```python
from build123d import *

# Parameters (mm, degrees)
BOSS_EXTRUDE1_DEPTH = 21
CHAMFER1_SIZE       = 0.5


with BuildPart() as part:
    # Sketch1 → Boss-Extrude1 (new body)
    with BuildSketch(Plane(origin=(0, 0, 0), x_dir=(1, 0, 0), z_dir=(0, 1, 0))):
        Polygon((4.041451884, 0), (2.020725942, 3.5), (-2.020725942, 3.5), (-4.041451884, 0), (-2.020725942, -3.5), (2.020725942, -3.5), align=None)
    extrude(amount=BOSS_EXTRUDE1_DEPTH)

    # Sketch2 → Cut-Revolve1 (revolve, cut)
    with BuildSketch(Plane.XY, mode=Mode.PRIVATE) as cut_revolve1_sk:
        Polygon((-1, 1.985640646), (-1, 21.445867252), (0, 21.445867252), (0, 0), (-0.2, 0), (-0.2, 0.6), align=None)
        Polygon((-3, 22.847292178), (-3, 6.770566956), (-2.5, 6.5), (-2.5, 5), (-6.012196156, 5), (-6.012196156, 2), (-1.654700538, 2), (-0.5, 0), (-0.5, -1.473098258), (-7.184398373, -1.473098258), (-7.184398373, 22.847292178), align=None)
    revolve(cut_revolve1_sk.sketch.rotate(Axis((0, 22.126511162, 0), (0, -1, 0)), 270), axis=Axis((0, 22.126511162, 0), (0, -1, 0)), mode=Mode.SUBTRACT)

    # Chamfer1
    chamfer1_edges = [part.edges().sort_by_distance(p)[0] for p in [
        (0, 21, -1),
        (0, 21, -3),
    ]]
    chamfer(chamfer1_edges, length=CHAMFER1_SIZE)


solid = part.part
```
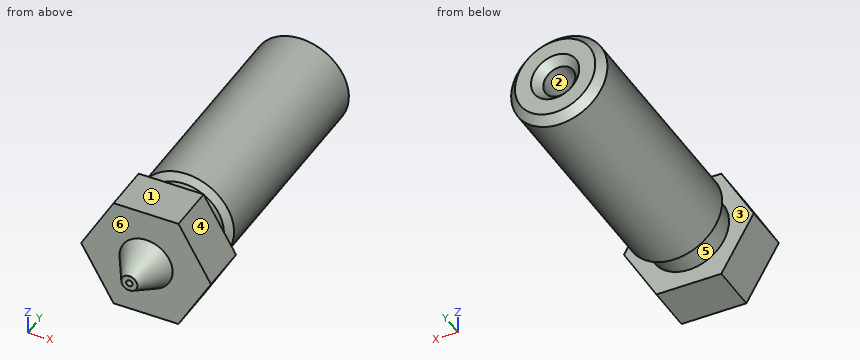
Could you check a few things on this model? Use its own coordinates, in mm. Face numbers are marked on the shaded views. A direction names the side the tool comes from. Round coordinates to 2 decimals unless told otherwise and drop trailing zeros. Write each loop counter-clockwise with the first axis right and the second up, starting at its lowest first coordinate (ties: lowest second). Pieces come first, ordered by that corner, then holes.
(1) Suppose I cut it at A-A on x = 0. Write out the boundary of the cut face in (y, z), and give its area (3 significant figures).
Findings below:
outline: (0, -0.5) - (2, -1.65) - (2, -3.5) - (5, -3.5) - (5, -2.5) - (6.5, -2.5) - (6.77, -3) - (20.5, -3) - (21, -2.5) - (21, -1.5) - (20.5, -1) - (1.99, -1) - (0.6, -0.2) - (0, -0.2) - close; (0, 0.2) - (0.6, 0.2) - (1.99, 1) - (20.5, 1) - (21, 1.5) - (21, 2.5) - (20.5, 3) - (6.77, 3) - (6.5, 2.5) - (5, 2.5) - (5, 3.5) - (2, 3.5) - (2, 1.65) - (0, 0.5) - close
area: 79.2 mm2
(2) Which directions (+Z, -Z, +X, -X, +Y, -Y) give clear straight access to the entire face, cutting with the end or side of a thin tool? Please do the marked faces 1, 2 and 3.
Findings below:
face 1: +Z, +X, -X, +Y, -Y
face 2: +Y
face 3: none
(3) Suppose I cut it at B-B on y = 14.75. Write out the boundary of the cut face in (x, z).
Findings below:
outline: circle Ø6 at (0, 0); hole circle Ø2 at (0, 0)
(4) If I drill on probe 1 along X at (y, z) = (16.75, 0); probe 2 along Z at (x, y) = (-0.25, 15.5); probe 3 along Y at (x, z) = (-1, -3), over which ranges is the centre line in solid material (lowest first)?
Findings below:
probe 1: x = -3 to -1, 1 to 3
probe 2: z = -2.99 to -0.97, 0.97 to 2.99
probe 3: y = 2 to 5
(5) Thinking about a two-plate mould opening in Y: for the marked faces 4, 5 and 6, which applies, +Y half, -Y half, draft (parallel to the pull), parting line (faces both ways), or undercut?
Findings below:
face 4: draft
face 5: undercut
face 6: -Y half
(6) For pin 1 (1.2 mm diameter, centred on x = 0, z = 0, fed in from +Y); pin 2 (1 mm diameter, centred on x = -2, z = -0.5, fed in from -Y); pin 3 (4 mm diameter, centred on x = -2.5, y = 13.5, fed in from +Z); pin 4 (3 mm diameter, centred on x = -0.5, z = 1, fed in from +Y), each with a flat end and sliding along its axis, tell me the tip position at first contact or that it passes through.
Findings below:
pin 1: stops at y = 1.29
pin 2: stops at y = 1.84
pin 3: stops at z = 2.96
pin 4: stops at y = 21
